The listing builds one solid part. Answer for the finished solid, in the listing's coordinates (mm). Round coordinates to 2 decimals unless told otherwise and drop trailing zeros. Order: outer loops, then holes, each group sorted by start corner. A loop starts at its lowest first (then second) coordinate and runs counter-clockwise, first axis right, second up. Notation, with made-up numbers: (12.5, -15.75) -> (45.5, -15.75) arc R18 cw to (45.5, -8.75) -> close; hole circle Ø10 at (70, 18.5). An arc over 180 degrees is marked (long way). Return JSON: item names as keys, results as strings. Group by question number.
(1) The part is cut by section A-A (z = 39). Determine the outline of the cut face in (x, y), plus the area to 3 significant figures.
(2) Determine the mould class of faces 1 (the face through (-26.159, -25.044, 47.658)), 2 (the face through (-7.34, -25.04, 17.03)), 3 (the face through (4.302, -25.044, 27.288)) for opening direction Z: +Z half, -Z half, draft (parallel to the pull), parting line (faces both ways), or undercut.
(3) Each of these flat-tipped pins is pushed along its axis until it touches: pin 1 (2 mm diameter, centred on x = -25, y = -30.5, fed in from +Z); pin 2 (5 mm diameter, centred on y = -14, z = 38.5, fed in from +X); pin 3 (2 mm diameter, centred on y = -16.5, z = 8, fed in from +X). Where does it stop, or does it pass through?
(4) The part is cut by section B-B (x = -32). Determine the outline of the cut face in (y, z).
(5) Consider line 1 (Z direction, x = -10.5, y = -34); line 2 (X direction, y = -26.5, z = 25); line 3 (Z direction, x = -6.5, y = -24). Determine where each line is inside the solid, lowest interval first. Write a range as [from, to].
(6) The part is cut by section C-C (y = -43.5). Count the separate pieces of the cut face and the enclosed holes in it, plus the area to 3 significant figures.
(7) The part is cut by section D-D (z = -8.5). Determine the outline of the cut face in (x, y).
from build123d import *

# Parameters (mm, degrees)
F1_DEPTH = 50.8
F2_W     = 6.985
F2_H     = 2.8702
F3_DEPTH = 50.8
F4_R     = 3.81
F5_DEPTH = 50.8


with BuildPart() as f1:
    # F0 (on Front) → F1 (new body)
    with BuildSketch(Plane.XZ):
        Polygon((-33.22611, 46.59294), (-47.547709, 41.43716), (-60.341675, 37.236158), (-75.618044, 28.643196), (-55.185895, 2.291456), (-28.643198, 12.984917), (-6.683412, -5.919594), (15.085417, -14.894464), (20.432146, -10.311551), (12.030142, -5.919594), (7.230051, -1.85285), (2.563801, 2.100501), (-1.718592, 5.72864), (-4.279601, 9.668654), (-8.108484, 15.559242), (-9.691619, 17.994835), (-10.605306, 19.400507), (-16.613055, 28.643196), (-6.683412, 28.643196), (-2.100501, 28.643196), (1.909546, 28.643196), (4.804504, 28.643196), (6.855496, 28.643196), (8.906488, 28.643196), (10.957481, 28.643196), (13.034425, 28.643196), (15.085417, 28.643196), (20.432146, 28.643196), (25.340278, 29.170681), (30.457475, 29.720634), (34.531654, 30.158492), (35.521915, 30.55086), (39.607522, 32.169688), (44.683389, 34.180883), (40.673338, 44.301476), (28.834153, 48.693441), (-19.28642, 48.693441), align=None)
        Polygon((44.683389, 25.969833), (44.683389, 34.180883), (39.607522, 32.169688), align=None)
        Polygon((39.607522, 25.969833), (39.607522, 32.169688), (35.521915, 30.55086), align=None)
        Polygon((35.521915, 24.251241), (35.521915, 30.55086), (34.531654, 30.158492), (30.457475, 29.720634), align=None)
        Polygon((12.030142, -5.919594), (20.432146, -10.311551), (21.768831, -4.201002), align=None)
        Polygon((7.230051, -1.85285), (12.030142, -5.919594), (12.030142, 0), align=None)
        Polygon((30.457475, 23.487423), (30.457475, 29.720634), (25.340278, 29.170681), align=None)
        Polygon((2.563801, 2.100501), (7.230051, -1.85285), (7.230051, 2.100501), align=None)
        Polygon((26.12297, 21.887899), (25.340278, 29.170681), (20.432146, 28.643196), align=None)
        Polygon((-1.718592, 5.72864), (2.563801, 2.100501), (1.819311, 6.319278), align=None)
        Polygon((20.432146, 23.487423), (20.432146, 28.643196), (15.085417, 28.643196), align=None)
        Polygon((-4.279601, 9.668654), (-1.718592, 5.72864), (-1.718592, 10.120597), align=None)
        Polygon((14.093683, 25.969833), (15.085417, 28.643196), (13.034425, 28.643196), align=None)
        Polygon((-8.108484, 15.559242), (-4.279601, 9.668654), (-4.279601, 13.557781), align=None)
        Polygon((12.030142, 25.936006), (13.034425, 28.643196), (10.957481, 28.643196), align=None)
        Polygon((-9.691619, 17.994835), (-8.108484, 15.559242), (-6.545077, 18.550107), align=None)
        Polygon((9.965747, 25.969833), (10.957481, 28.643196), (8.906488, 28.643196), align=None)
        Polygon((-10.605306, 19.400507), (-9.691619, 17.994835), (-8.108484, 21.023442), align=None)
        Polygon((7.914755, 25.969833), (8.906488, 28.643196), (6.855496, 28.643196), align=None)
        Polygon((5.863763, 25.969833), (6.855496, 28.643196), (4.804504, 28.643196), align=None)
        Polygon((3.812771, 25.969833), (4.804504, 28.643196), (1.909546, 28.643196), align=None)
        Polygon((-2.100501, 28.643196), (-6.683412, 28.643196), (-3.092235, 25.969833), align=None)
        Polygon((0.917812, 25.969833), (1.909546, 28.643196), (-2.100501, 28.643196), align=None)
    extrude(amount=F1_DEPTH)

    # F2 (on face) → F3 (cut)
    with BuildSketch(Plane.XZ.offset(50.8)):
        with Locations((22.857464, 41.59747)):
            Rectangle(F2_W, F2_H)
    extrude(amount=-F3_DEPTH, mode=Mode.SUBTRACT)

    # F4 (on face) → F5 (cut)
    with BuildSketch(Plane.XZ.offset(50.8)):
        with Locations((-8.494654, 40.573284)):
            Circle(F4_R)
    extrude(amount=-F5_DEPTH, mode=Mode.SUBTRACT)


solid = f1.part
Answer below:
{
 "1": {"outline": "(-54.97, -50.8) -> (-11.96, -50.8) -> (-11.96, 0) -> (-54.97, 0) -> close; (-5.02, -50.8) -> (42.77, -50.8) -> (42.77, 0) -> (-5.02, 0) -> close", "area": "4,610 mm²"},
 "2": {"face 1": "+Z half", "face 2": "undercut", "face 3": "undercut"},
 "3": {"pin 1": "stops at z = 47.98", "pin 2": "stops at x = 43.96", "pin 3": "stops at x = -1.72"},
 "4": {"outline": "(-50.8, 11.63) -> (0, 11.63) -> (0, 46.78) -> (-50.8, 46.78) -> close"},
 "5": {"line 1": "z = [-2.63, 19.47], [28.64, 37.33], [43.81, 48.69]", "line 2": "x = [-72.79, -14.24], [18.86, 20.43], [23.5, 25.79], [29.1, 30.46], [34.83, 35.52]", "line 3": "z = [-6, 14.72], [28.51, 37.33], [43.82, 48.69]"},
 "6": {"separate pieces": "1", "enclosed holes": "2", "area": "3,570 mm²"},
 "7": {"outline": "(-0.42, -50.8) -> (20.83, -50.8) -> (20.83, 0) -> (-0.42, 0) -> close"}
}
